```python
from build123d import *
from build123d.topology import SkipClean

# Parameters (mm, degrees)
BOSS_EXTRUDE1_DEPTH      = 3.175
SKETCH2_W                = 73.3096723
SKETCH2_H                = 3.175
BOSS_EXTRUDE2_DEPTH      = 33.528
BOSS_EXTRUDE3_START      = 7.8105
BOSS_EXTRUDE3_DEPTH      = 7.8105
SKETCH4_W                = 3.175
SKETCH4_H                = 33.528
BOSS_EXTRUDE4_DEPTH      = 2.98186385
SKETCH5_W                = 3.175
SKETCH5_H                = 33.528
BOSS_EXTRUDE5_DEPTH      = 2.98186385
SKETCH6_W                = 79.2734
SKETCH6_H                = 10.9855
BOSS_EXTRUDE6_DEPTH      = 13.843
SKETCH7_W                = 29.972
SKETCH7_H                = 7.8105
CUT_EXTRUDE1_DEPTH       = 8.763
SKETCH8_W                = 29.972
SKETCH8_H                = 7.8105
CUT_EXTRUDE2_DEPTH       = 8.763
BOSS_EXTRUDE7_DEPTH      = 7.8105
CUT_EXTRUDE3_DEPTH       = 97.500739167
SKETCH11_W               = 30.353
SKETCH11_H               = 18.796
HOLE1_D                  = 5.08
HOLE1_CBORE_D            = 11.811
HOLE1_CBORE_DEPTH        = 14.143710789
M7_CLEARANCE_HOLE1_D     = 7.8232
M7_CLEARANCE_HOLE1_DEPTH = 10.9855
M7_CLEARANCE_HOLE2_D     = 7.8232
M7_CLEARANCE_HOLE2_DEPTH = 10.9855
FILLET1_R                = 1.57988
FILLET2_R                = 2.794


with BuildPart() as part:
    # Sketch1 → Boss-Extrude1 (new body)
    with BuildSketch(Plane(origin=(0, 0, -1.5875), x_dir=(-1, 0, 0), z_dir=(0, 0, -1))):
        with BuildLine():
            Line((-36.65483615, 47.371), (36.65483615, 47.371))
            ThreePointArc((36.65483615, 47.371), (0, 85.953679717), (-36.65483615, 47.371))
        make_face()
    extrude(amount=-BOSS_EXTRUDE1_DEPTH)

    # Sketch2 → Boss-Extrude2 (add)
    with BuildSketch(Plane.XZ.offset(-47.371)):
        Rectangle(SKETCH2_W, SKETCH2_H)
    extrude(amount=BOSS_EXTRUDE2_DEPTH)

    # Sketch3 → Boss-Extrude3 (add)
    with SkipClean():  # the faces are left unmerged after this step: merging them gives an invalid solid
        with BuildSketch(Plane(origin=(0, 0, -1.5875), x_dir=(-1, 0, 0), z_dir=(0, 0, -1)).offset(BOSS_EXTRUDE3_START)):
            with BuildLine():
                Line((9.6647, 13.843), (-9.6647, 13.843))
                ThreePointArc((-9.6647, 13.843), (0, 85.953679717), (9.6647, 13.843))
            make_face()
        extrude(amount=-BOSS_EXTRUDE3_DEPTH)

    # Sketch4 → Boss-Extrude4 (add)
    with SkipClean():  # the faces are left unmerged after this step: merging them gives an invalid solid
        with BuildSketch(Plane.ZY.offset(36.65483615)):
            with Locations((0, 30.607)):
                Rectangle(SKETCH4_W, SKETCH4_H)
        extrude(amount=BOSS_EXTRUDE4_DEPTH)

    # Sketch5 → Boss-Extrude5 (add)
    with SkipClean():  # the faces are left unmerged after this step: merging them gives an invalid solid
        with BuildSketch(Plane(origin=(36.65483615, 0, 0), x_dir=(0, 0, -1), z_dir=(1, 0, 0))):
            with Locations((0, 30.607)):
                Rectangle(SKETCH5_W, SKETCH5_H)
        extrude(amount=BOSS_EXTRUDE5_DEPTH)

    # Sketch6 → Boss-Extrude6 (add)
    with SkipClean():  # the faces are left unmerged after this step: merging them gives an invalid solid
        with BuildSketch(Plane.XZ.offset(-13.843)):
            with Locations((0, -3.90525)):
                Rectangle(SKETCH6_W, SKETCH6_H)
        extrude(amount=BOSS_EXTRUDE6_DEPTH)

    # Sketch7 → Cut-Extrude1 (cut)
    with SkipClean():  # the faces are left unmerged after this step: merging them gives an invalid solid
        with BuildSketch(Plane(origin=(0, 13.843, 0), x_dir=(-1, 0, 0), z_dir=(0, 1, 0))):
            with Locations((-24.6507, -5.49275)):
                Rectangle(SKETCH7_W, SKETCH7_H)
        extrude(amount=-CUT_EXTRUDE1_DEPTH, mode=Mode.SUBTRACT)

    # Sketch8 → Cut-Extrude2 (cut)
    with SkipClean():  # the faces are left unmerged after this step: merging them gives an invalid solid
        with BuildSketch(Plane(origin=(0, 13.843, 0), x_dir=(-1, 0, 0), z_dir=(0, 1, 0))):
            with Locations((24.6507, -5.49275)):
                Rectangle(SKETCH8_W, SKETCH8_H)
        extrude(amount=-CUT_EXTRUDE2_DEPTH, mode=Mode.SUBTRACT)

    # Sketch9 → Boss-Extrude7 (add)
    with SkipClean():  # the faces are left unmerged after this step: merging them gives an invalid solid
        with BuildSketch(Plane.XY.offset(1.5875)):
            with BuildLine():
                Line((9.6647, 13.843), (9.6647, 5.08))
                Line((9.6647, 5.08), (39.6367, 5.08))
                Line((39.6367, 5.08), (39.6367, 0))
                Line((39.6367, 0), (-39.6367, 0))
                Line((-39.6367, 0), (-39.6367, 5.08))
                Line((-39.6367, 5.08), (-9.6647, 5.08))
                Line((-9.6647, 5.08), (-9.6647, 13.843))
                ThreePointArc((-9.6647, 13.843), (0, 85.953679717), (9.6647, 13.843))
            make_face()
        extrude(amount=BOSS_EXTRUDE7_DEPTH)

    # Sketch10 → Cut-Extrude3 (cut, through all)
    with SkipClean():  # the faces are left unmerged after this step: merging them gives an invalid solid
        with BuildSketch(Plane.XY.offset(9.398)):
            with BuildLine():
                ThreePointArc((-29.562039749, 71.003748808), (-25.123016493, 71.679265301), (-24.4475, 67.240242044))
                ThreePointArc((-24.4475, 67.240242044), (0, 79.603679717), (24.4475, 67.240242044))
                ThreePointArc((24.4475, 67.240242044), (25.123016493, 71.679265301), (29.562039749, 71.003748808))
                ThreePointArc((29.562039749, 71.003748808), (0, 85.953679717), (-29.562039749, 71.003748808))
            make_face()
        extrude(amount=-CUT_EXTRUDE3_DEPTH, mode=Mode.SUBTRACT)

    # Sketch11 → Cut-Revolve1 (revolve, cut)
    with SkipClean():  # the faces are left unmerged after this step: merging them gives an invalid solid
        with BuildSketch(Plane.XZ.offset(-49.250679717)):
            with Locations((15.1765, 0)):
                Rectangle(SKETCH11_W, SKETCH11_H)
        revolve(axis=Axis((0, 49.250679717, 9.398), (0, 0, -1)), mode=Mode.SUBTRACT)

    # Hole1 (through all)
    with Locations(Plane(origin=(0, 19.477710789, 0), x_dir=(1, 0, 0), z_dir=(0, 1, 0))):
        with Locations((0, 0)):
            CounterBoreHole(HOLE1_D / 2, HOLE1_CBORE_D / 2, HOLE1_CBORE_DEPTH)

    # M7 Clearance Hole1
    with Locations(Plane(origin=(0, 0, -1.5875), x_dir=(-1, 0, 0), z_dir=(0, 0, -1))):
        with Locations((30.2387, 13.208)):
            Hole(M7_CLEARANCE_HOLE1_D / 2, depth=M7_CLEARANCE_HOLE1_DEPTH)

    # M7 Clearance Hole2
    with Locations(Plane.XY.offset(1.5875)):
        with Locations((30.2387, 13.208)):
            Hole(M7_CLEARANCE_HOLE2_D / 2, depth=M7_CLEARANCE_HOLE2_DEPTH)

    # Fillet1
    # the kernel refuses this fillet: 1.57988 mm, written as the material it takes off along each edge
    with BuildSketch(Plane(origin=(-39.6367, 13.843, -1.5875), x_dir=(1, 0, 0), z_dir=(0, 1, 0)), Plane(origin=(39.6367, 51.3207, -1.5875), x_dir=(-1, 0, 0), z_dir=(0, -1, 0)), Plane(origin=(-39.6367, 51.3207, 1.5875), x_dir=(1, 0, 0), z_dir=(0, -1, 0))) as fillet1_piece_1:
        with BuildLine():
            CenterArc((FILLET1_R, -FILLET1_R), FILLET1_R, 90, 90)
            Line((0, -FILLET1_R), (0, 0))
            Line((0, 0), (FILLET1_R, 0))
        make_face()
    extrude(amount=37.4777, mode=Mode.SUBTRACT)
    with BuildSketch(Plane(origin=(39.6367, 13.843, 1.5875), x_dir=(0, 0, -1), z_dir=(0, 1, 0))) as fillet1_piece_2:
        with BuildLine():
            CenterArc((FILLET1_R, FILLET1_R), FILLET1_R, 180, 90)
            Line((0, FILLET1_R), (0, 0))
            Line((0, 0), (FILLET1_R, 0))
        make_face()
    extrude(amount=37.4777, mode=Mode.SUBTRACT)
    with BuildSketch(Plane(origin=(-39.6367, 13.843, 1.5875), x_dir=(1, 0, 0), z_dir=(0, -1, 0)), Plane(origin=(39.6367, 13.843, 1.5875), x_dir=(0, 0, -1), z_dir=(0, -1, 0))) as fillet1_piece_3:
        with BuildLine():
            CenterArc((FILLET1_R, -FILLET1_R), FILLET1_R, 90, 90)
            Line((0, -FILLET1_R), (0, 0))
            Line((0, 0), (FILLET1_R, 0))
        make_face()
    extrude(amount=8.763, mode=Mode.SUBTRACT)
    with BuildSketch(Plane(origin=(39.6367, 13.843, -1.5875), x_dir=(0, 0, 1), z_dir=(0, -1, 0)), Plane(origin=(-39.6367, 13.843, -1.5875), x_dir=(1, 0, 0), z_dir=(0, -1, 0))) as fillet1_piece_4:
        with BuildLine():
            CenterArc((FILLET1_R, FILLET1_R), FILLET1_R, 180, 90)
            Line((0, FILLET1_R), (0, 0))
            Line((0, 0), (FILLET1_R, 0))
        make_face()
    extrude(amount=8.763, mode=Mode.SUBTRACT)

    # Fillet2
    fillet2_edges = [part.edges().sort_by_distance(p)[0] for p in [
        (-39.6367, 2.54, 9.398),
        (39.6367, 2.54, 9.398),
        (-39.6367, 2.54, -9.398),
        (39.6367, 2.54, -9.398),
    ]]
    fillet(fillet2_edges, radius=FILLET2_R)


solid = part.part
```
The listing builds one solid part. Answer for the finished solid, in the listing's coordinates (mm). A direction names the side the tool comes from. Give positions to 0.01 mm unless a question says otherwise; leave off trailing zeros. Order: outer loops, then holes, each group sorted by start corner. A loop starts at its lowest first (then second) coordinate and runs counter-clockwise, first axis right, second up. Notation, with made-up numbers: (65, -36.5) - (74, -36.5) arc R26 ccw to (74, -13.5) - close; hole circle Ø8 at (-38.5, 45.25). An arc over 180 degrees is marked (long way). Answer in a Markdown table with one row per item. Add a question column.
Q1. The part is cut by section B-B (x = 0). Determine the outline of the cut face in (y, z), then the cut area to 3 significant figures.
Q2. Which of the six approach directions +Z, -Z, +X, -X, +Y, -Y give full straight-line access (tool end or side, diameter ignored) to faces 4 (the flat face through (-24, 5.08, -6)), 5 (the flat face through (24, 5.08, 6)), 6 (the flat face through (27, 17, -1.588))?
Q3. Given P1, Ø6, axis at y = 56, z = 6.5, coming from the +X side; P2, Ø8, axis at x = 0, z = 0, coming from the +Y side; P3, Ø5, axis at y = 58.5, z = -6, coming from the +X side; P4, Ø8.5, axis at y = 8, z = -7, coming from the -X side, each flat-ended and moving along its own axis, determine where each tip first touches the part or whether it passes through.
Q4. For a pull along Z with two mould halves and no side action, classify faces 1 (the cylindrical face through (-38.8, 2.5, -8.6)), 2 (the flat face through (39.637, 3, 0)), 3 (the cylindrical face through (-4.69, 12.5, 3.59)) as released by +Z, released by -Z, zero draft, split by the parting line, or undercut.
Q5. Find the intervals of material crossed by line 1 along Z through (x, y) = (0, 2.75); line 2 along Z through (x, y) = (0, 10.75); line 3 along Y through (x, z) = (-31, -6.75), in increasing order. Write a range as [from, to].
Q6. The part is cut by section C-C (x = -28). Determine the outline of the cut face in (y, z), then the cut area to 3 significant figures.
Determined:
| question | item | result |
|---|---|---|
| 1 | outline | (0, -9.4) - (18.9, -9.4) - (18.9, -5.91) - (5.33, -5.91) - (5.33, -2.54) - (0, -2.54) - close; (0, 2.54) - (5.33, 2.54) - (5.33, 5.91) - (18.9, 5.91) - (18.9, 9.4) - (0, 9.4) - close |
| 1 | area | 168 mm² |
| 2 | face 4 | -Z, -X |
| 2 | face 5 | +Z, +X |
| 2 | face 6 | -Z, +X |
| 3 | P1 | stops at x = 36.51 |
| 3 | P2 | stops at y = 5.33 |
| 3 | P3 | stops at x = 36.08 |
| 3 | P4 | stops at x = -39.64 |
| 4 | face 1 | released by -Z |
| 4 | face 2 | zero draft |
| 4 | face 3 | undercut |
| 5 | line 1 | z = [-9.4, -2.54], [2.54, 9.4] |
| 5 | line 2 | z = [-9.4, -5.91], [5.91, 9.4] |
| 5 | line 3 | y = [0, 5.08], [29.6, 68.9] |
| 6 | outline | (0, -9.4) - (5.08, -9.4) - (5.08, -1.59) - (10, -1.59) - (10, 1.59) - (5.08, 1.59) - (5.08, 9.4) - (0, 9.4) - close; (16.42, -1.59) - (25.52, -1.59) - (25.52, -9.4) - (37.53, -9.4) - (37.53, 9.4) - (25.52, 9.4) - (25.52, 1.59) - (16.42, 1.59) - close; (60.97, -9.4) - (72.14, -9.4) - (72.14, 9.4) - (60.97, 9.4) - close |
| 6 | area | 576 mm² |
